For this review, take the finished solid that the model builds, in its own axes (mm). Face numbers are marked on the shaded views. A direction names the side the tool comes from. Coordinates: 2 decimals unless noted, no trailing zeros. Order: outer loops, then holes, each group sorted by start corner. A loop starts at its lowest first (then second) coordinate and runs counter-clockwise, first axis right, second up. Notation, with made-up numbers: (2, 9.25) -> (29, 9.25) arc R10 ccw to (29, 21.25) -> close; hole circle Ø4 at (85.25, 28). An arc over 180 degrees is marked (long way). Return JSON: item names as keys, results as strings. Group by question number.
Item 1: Draft analysis for pull direction X (two halves, no side actions). For the marked faces 5, 6, 7 and 8, state which applies: +X half, -X half, draft (parallel to the pull), parting line (faces both ways), or undercut.
Item 2: Machinability: for the marked faces 1, 2, 3 and 4, which of the approach directions +Z, -Z, +X, -X, +Y, -Y give a long, thin tool a straight path to every point of the face, cutting with its end or side? Answer none if there is none.
Item 3: Take a section at D-D (y = -71). Write out the cut boundary in (x, z), then the cut area to 3 significant figures.
Item 4: Take a section at A-A (x = 72). Write out the cut boundary in (y, z).
Item 5: Take a section at B-B (z = 931). Write out the cut boundary in (x, y).
Item 6: For line 1 along X through (y, z) = (-131.5, 1384.5); line 2 along Z through (x, y) = (322.5, -125); line 3 along Y through (x, z) = (278, 123), list the stretches that pass through material, from the lowest coordinate up.
Item 7: Insertion check: pin 1 (20 mm diameter, centred on x = 336.5, y = -148.5, fed in from -Z); pin 2 (3 mm diameter, centred on x = 102, z = 713.5, fed in from -Y); pin 3 (4 mm diameter, centred on x = 443, y = -19, fed in from +Z). Each pin has a flat end and moves straight along its axis. Give the tip position at first contact, or say it passes through.
Item 8: Take a section at C-C (x = 621). Count the separate pieces of the cut face and the enclosed holes in it, then the cut area to 3 significant figures.
```python
from build123d import *

# Parameters (mm, degrees)
F1_DEPTH  = 18
F3_W      = 740
F3_H      = 1382
F3_W_2    = 500
F3_H_2    = 200
F3_W_3    = 280
F3_H_3    = 40
F4_DEPTH  = 18
F7_DEPTH  = 18
F9_W      = 740
F9_H      = 160
F10_DEPTH = 18
F12_W     = 740
F12_H     = 410
F13_DEPTH = 18
F15_W     = 740
F15_H     = 225
F15_H_2   = 75
F16_DEPTH = 18
F17_R     = 4.9999


# Not quite as in the source:
# - a fillet or chamfer is up to 0.001 mm smaller than in the source, because OpenCascade refuses the exact size


with BuildPart() as f1:
    # F0 (on Right) → F1 (new body)
    with BuildSketch(Plane.YZ):
        with BuildLine():
            Line((-435, 0), (0, 0))
            Line((0, 0), (0, 1850))
            Line((0, 1850), (-100, 1850))
            ThreePointArc((-100, 1850), (-153.033008589, 1828.033008589), (-175, 1775))
            Line((-175, 1775), (-175, 441.066017178))
            ThreePointArc((-175, 441.066017178), (-180.7090350617, 412.3647597506), (-196.966991411, 388.033008589))
            Line((-196.966991411, 388.033008589), (-413.033008589, 171.966991411))
            ThreePointArc((-413.033008589, 171.966991411), (-429.2909649383, 147.6352402494), (-435, 118.933982822))
            Line((-435, 118.933982822), (-435, 0))
        make_face()
    extrude(amount=F1_DEPTH)

    # F3 (on offset) → F4 (join)
    with BuildSketch(Plane.XZ.offset(160)):
        with Locations((388, 719)):
            Rectangle(F3_W, F3_H)
        with Locations((388, 1005)):
            Rectangle(F3_W_2, F3_H_2, mode=Mode.SUBTRACT)
        with Locations((388, 1180)):
            Rectangle(F3_W_3, F3_H_3, mode=Mode.SUBTRACT)
    extrude(amount=-F4_DEPTH)

    # F6 (on offset) → F7 (join)
    with BuildSketch(Plane.YZ.offset(758)):
        with BuildLine():
            Line((-435, 0), (0, 0))
            Line((0, 0), (0, 1850))
            Line((0, 1850), (-100, 1850))
            ThreePointArc((-100, 1850), (-153.033008589, 1828.033008589), (-175, 1775))
            Line((-175, 1775), (-175, 441.066017178))
            ThreePointArc((-175, 441.066017178), (-180.7090350617, 412.3647597506), (-196.966991411, 388.033008589))
            Line((-196.966991411, 388.033008589), (-413.033008589, 171.966991411))
            ThreePointArc((-413.033008589, 171.966991411), (-429.2909649383, 147.6352402494), (-435, 118.933982822))
            Line((-435, 118.933982822), (-435, 0))
        make_face()
    extrude(amount=F7_DEPTH)

    # F9 (on offset) → F10 (join)
    with BuildSketch(Plane.XY.offset(1410)):
        with Locations((388, -90)):
            Rectangle(F9_W, F9_H)
    extrude(amount=F10_DEPTH)

    # F12 (on offset) → F13 (join)
    with BuildSketch(Plane(origin=(0, -10, 0), x_dir=(-1, 0, 0), z_dir=(0, 1, 0))):
        with Locations((-388, 1633)):
            Rectangle(F12_W, F12_H)
    extrude(amount=-F13_DEPTH)

    # F15 (on offset) → F16 (join)
    with BuildSketch(Plane(origin=(0, 0, 28), x_dir=(1, 0, 0), z_dir=(0, 0, -1))):
        with Locations((388, 122.5)):
            Rectangle(F15_W, F15_H)
        with Locations((388, 392.5)):
            Rectangle(F15_W, F15_H_2)
    extrude(amount=F16_DEPTH)

    # F17 (radius 5 in the source; OpenCascade refuses exactly that, so slightly less here)
    f17_edges = [f1.edges().sort_by_distance(p)[0] for p in [
        (388, -170, 1428),
        (388, -170, 1410),
        (758, -175, 1108.033009),
        (776, -175, 1108.033009),
        (388, -28, 1838),
        (388, -10, 1838),
        (18, -50, 1850),
        (0, -50, 1850),
        (388, -235, 28),
        (388, -355, 28),
        (388, -430, 28),
        (388, -430, 10),
        (388, -235, 10),
    ]]
    fillet(f17_edges, radius=F17_R)


solid = f1.part
```
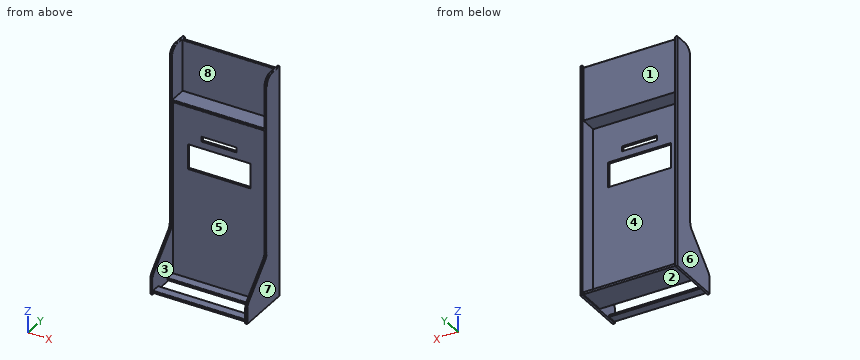
Findings below:
{
 "1": {"face 5": "undercut", "face 6": "-X half", "face 7": "+X half", "face 8": "undercut"},
 "2": {"face 1": "+Z, -Z, +Y", "face 2": "-Z, +Y, -Y", "face 3": "none", "face 4": "+Y"},
 "3": {"outline": "(0, 0) -> (18, 0) -> (18, 10) -> (758, 10) -> (758, 0) -> (776, 0) -> (776, 1845) arc R5 ccw to (771, 1850) -> (763, 1850) arc R5 ccw to (758, 1845) -> (758, 1428) -> (18, 1428) -> (18, 1845) arc R5 ccw to (13, 1850) -> (5, 1850) arc R5 ccw to (0, 1845) -> close; hole (18, 28) -> (758, 28) -> (758, 1410) -> (18, 1410) -> close", "area": "93,200 mm2"},
 "4": {"outline": "(-430, 15) arc R5 ccw to (-425, 10) -> (-355, 10) -> (-355, 23) arc R5 ccw to (-360, 28) -> (-425, 28) arc R5 ccw to (-430, 23) -> close; (-235, 15) arc R5 ccw to (-230, 10) -> (-10, 10) -> (-10, 28) -> (-142, 28) -> (-142, 1410) -> (-10, 1410) -> (-10, 1833) arc R5 ccw to (-15, 1838) -> (-23, 1838) arc R5 ccw to (-28, 1833) -> (-28, 1428) -> (-165, 1428) arc R5 ccw to (-170, 1423) -> (-170, 1415) arc R5 ccw to (-165, 1410) -> (-160, 1410) -> (-160, 28) -> (-230, 28) arc R5 ccw to (-235, 23) -> close"},
 "5": {"outline": "(0, -170) arc R5 ccw to (5, -175) -> (13, -175) arc R5 ccw to (18, -170) -> (18, -160) -> (138, -160) -> (138, -142) -> (18, -142) -> (18, 0) -> (0, 0) -> close; (638, -160) -> (758, -160) -> (758, -170) arc R5 ccw to (763, -175) -> (771, -175) arc R5 ccw to (776, -170) -> (776, 0) -> (758, 0) -> (758, -142) -> (638, -142) -> close"},
 "6": {"line 1": "x = 0 to 18, 758 to 776", "line 2": "z = 10 to 28, 1410 to 1428", "line 3": "y = -160 to -142"},
 "7": {"pin 1": "stops at z = 10", "pin 2": "stops at y = -160", "pin 3": "stops at z = 1838"},
 "8": {"separate pieces": "3", "enclosed holes": "0", "area": "36,900 mm2"}
}
